Build history of the part. All positions in model axes, mm. A direction names the side the tool comes from. Give positions to 0.01 mm unless a question says otherwise; leave off trailing zeros. Loops run counter-clockwise (first coordinate to the right, second up) from the corner with the lowest first, then second, coordinate; pieces in that order, holes last.
1) 3-axis set-ups, long thin cutter, end or side, ignore diameter. For faces 1 (the flat face through (338, 25.4, 11)), 2 (the flat face through (338, 3.175, 11)): which of +Z, -Z, +X, -X, +Y, -Y reach the whole face in a straight line?
2) Band-saw the part on A-A on x = 155. List the corners of the cut face in (y, z) (3 decimals), then the cut area to 3 significant figures.
3) Wall check: line 1 (Y direction, x = 558.5, z = 2) (3 decimals); line 2 (Z direction, x = 63.5, y = 2.45) (3 decimals); line 3 (Z direction, x = 153.5, y = 13) (3 decimals). Give the ranges that are in metal, low to high.
4) Flat gauge pins, fed straight in: P1, Ø5, axis at x = 266.7, z = 12.7, coming from the -Y side; P2, Ø1.5, axis at x = 481, y = 10, coming from the -Z side (3 decimals). Where does each tip first touch, or does it go through?
5) Two-plate mould, pull along Y, no slides. Class faces 3 (the flat face through (338, 13, 22.225)), 4 (the flat face through (0, 12, 23)), 5 (the flat face through (338, 0, 11)): +Y half, -Y half, draft (parallel to the pull), parting line (faces both ways), or undercut.
6) Band-saw the part on B-B on y = 14. List the corners of the cut face in (x, z) (3 decimals).
Autodesk Inventor part; units mm, degrees
ref_plane "YZ Plane" through (0, 0, 0) normal (1, 0, 0) x (0, 1, 0)
ref_plane "XZ Plane" through (0, 0, 0) normal (0, 1, 0) x (-1, 0, 0)
ref_plane "XY Plane" through (0, 0, 0) normal (0, 0, 1) x (1, 0, 0)
sketch "Sketch1" plane through (0, 0, 0) normal (1, 0, 0) x (0, 1, 0)
  line L0 (0, 0) -> (0, 22.225)
  line L1 (3.175, 25.4) -> (22.225, 25.4)
  line L2 (25.4, 22.225) -> (25.4, 0)
  line L3 (22.225, 0) -> (22.225, 22.225)
  line L4 (22.225, 22.225) -> (3.175, 22.225)
  line L5 (3.175, 22.225) -> (3.175, 0)
  line L6 (0, 0) -> (3.175, 0)
  line L7 (22.225, 0) -> (25.4, 0)
  arc A0 (3.175, 25.4) -> (0, 22.225) centre (3.175, 22.225) ccw
  arc A1 (25.4, 22.225) -> (22.225, 25.4) centre (22.225, 22.225) ccw
  point P0 (0, 25.4)
  point P1 (25.4, 25.4)
  dimension "d0" = 25.4
  dimension "d2" = 25.4
  dimension "d3" = 90
  dimension "d4" = 25.4
  dimension "d5" = 90
  dimension "d6" = 3.175
  dimension "d7" = 3.175
extrude "Extrusion1" add sketch "Sketch1" along normal blind 685.8
sketch "Sketch2" plane through (0, 25.4, 22.225) normal (0, 1, 0) x (1, 0, 0)
  line L0 (0, 0) -> (0, 22.225)
  line L1 (0, 0) -> (685.8, 0)
  line L2 (685.8, 22.225) -> (685.8, 0)
  line L3 (0, 22.225) -> (685.8, 22.225)
  point P0 (12.7, 9.525)
  dimension "d10" = 12.7
  dimension "d11" = 12.7
hole "Hole1" at (12.7, 25.4, 12.7) direction (0, -1, 0) diameter 6.35 end through all
pattern_linear "Rectangular Pattern1" count 27 spacing 25.4 along (1, 0, 0) of "Hole1"
properties part number "c-channel"
Findings below:
1. face 1: +Z, -Z, +X, -X, +Y
1. face 2: -Z, +X, -X
2. outline: (0, 0) - (3.175, 0) - (3.175, 22.225) - (22.225, 22.225) - (22.225, 0) - (25.4, 0) - (25.4, 22.225) arc R3.175 ccw to (22.225, 25.4) - (3.175, 25.4) arc R3.175 ccw to (0, 22.225) - close
2. area: 217 mm2
3. line 1: y = 0 to 3.175, 22.225 to 25.4
3. line 2: z = 0 to 9.525, 15.875 to 25.316
3. line 3: z = 22.225 to 25.4
4. P1: passes through
4. P2: stops at z = 22.225
5. face 3: undercut
5. face 4: draft
5. face 5: -Y half
6. outline: (0, 22.225) - (685.8, 22.225) - (685.8, 25.4) - (0, 25.4) - close
